Autodesk Inventor part; units mm, degrees
ref_plane "YZ Plane" through (0, 0, 0) normal (1, 0, 0) x (0, 1, 0)
ref_plane "XZ Plane" through (0, 0, 0) normal (0, 1, 0) x (-1, 0, 0)
ref_plane "XY Plane" through (0, 0, 0) normal (0, 0, 1) x (1, 0, 0)
sketch "Sketch1" plane through (0, 0, 0) normal (1, 0, 0) x (0, 1, 0)
  circle A0 centre (0, 0) radius 1.9685
  dimension "d0" = 3.937
extrude "Extrusion1" add sketch "Sketch1" along normal blind 18.034
thread "Thread1"
sketch "Sketch2" plane through (0, 0, 0) normal (0, 1, 0) x (-1, 0, 0)
  line L0 (-18.034, 1.9685) -> (0, 1.9685)
  line L1 (0, 1.9685) -> (0, -1.9685)
  line L2 (0, -1.9685) -> (-18.034, -1.9685)
  line L3 (-18.034, -1.9685) -> (-18.034, 1.9685)
  circle A0 centre (-7.62, 6.9469) radius 6.223
  point P0 (0, 0)
  dimension "d6" = 7.62
  dimension "d7" = 4.9784
  dimension "d8" = 12.446
extrude "Extrusion2" cut sketch "Sketch2" along normal through all both and the other way through all contours A0 L0 | L0 A0
chamfer "Chamfer1" distance 0.3969 angle 45 1 edges at (18.034, -1.9685, 0)
properties part number "Screw Lock"
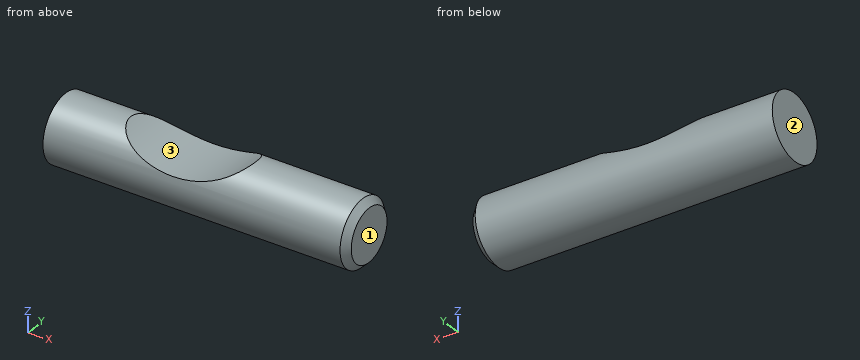
Geometry: final body of the model. Coordinates: model frame, mm. Face numbers are marked on the shaded views. Round coordinates to 2 decimals unless told otherwise and drop trailing zeros. Loops run counter-clockwise (first coordinate to the right, second up) from the corner with the lowest first, then second, coordinate; pieces in that order, holes last. Notation, with made-up numbers: (87, 5) -> (138, 5) arc R32 cw to (138, 31) -> close; hole circle Ø2 at (52.25, -32.75). An arc over 180 degrees is marked (long way). Use one line per item in the form item = value. Start each with the question number.
1) Section B-B on x = 12.75. Output: boundary loops of the cut face in (y, z), then the cut area to 3 significant figures.
2) Section C-C on x = 5. Output: boundary loops of the cut face in (y, z).
3) Line query: L1, parallel to Z at x = 3.25, y = 1.15; L2, parallel to Z at x = 3.25, y = -0.2; L3, parallel to X at y = -0.3, z = 1.3 (3 decimals). Output: solid intervals per line, ascending.
4) Draft query along X for the marked faces 1, 2 and 3. Return one class per face: released by +X, released by -X, zero draft, split by the parting line, or undercut.
5) Section A-A on y = 0. Output: boundary loops of the cut face in (x, z).
6) First-contact query: P1, Ø1, axis at x = 2, y = 1, coming from the -Z side. Flat tip, straight axial feed; report the tip coordinate or a pass-through.
Response:
q1.outline = circle Ø3.94 at (0, 0)
q1.area = 12.2 mm^2
q2.outline = (-1.48, 1.3) arc R1.97 ccw (long way) to (1.48, 1.3) -> close
q3.L1 = -1.6 to 1.6
q3.L2 = -1.96 to 1.96
q3.L3 = 0 to 5.005, 10.235 to 18.034
q4.face_1 = released by +X
q4.face_2 = released by -X
q4.face_3 = undercut
q5.outline = (0, -1.97) -> (17.64, -1.97) -> (18.03, -1.57) -> (18.03, 1.57) -> (17.64, 1.97) -> (11.35, 1.97) arc R6.22 cw to (3.89, 1.97) -> (0, 1.97) -> close
q6.P1 = -1.9
